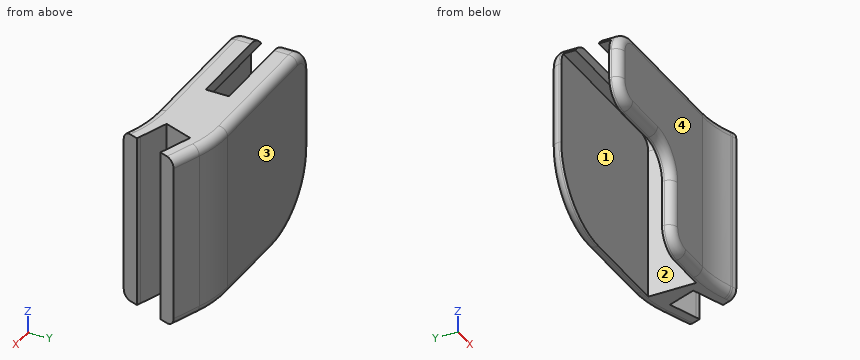
```python
from build123d import *

# Parameters (mm, degrees)
F0_W         = 30
F0_H         = 12
F1_DEPTH     = 30
F2_W         = 8.215
F2_H         = 28.15
F3_DEPTH     = 28
F4_W         = 5.3
F4_H         = 30
F5_DEPTH     = 5.3
F6_W         = 17
F6_H         = 17
F7_DEPTH     = 2.8
F8_DEPTH     = 0.75
F9_R         = 12
F10_T1_DEPTH = 32
F10_T3_DEPTH = 11.8925
F11_R        = 20
F12_R        = 5
F13_R        = 1.5
F14_R        = 2
F15_W        = 5.0863461345
F15_H        = 4
F15_W_2      = 14.4734603858
F16_DEPTH    = 30.0010001


# Not quite as in the source:
# - a fillet or chamfer that OpenCascade refuses, or shapes differently, is made with other operations: its cross-section is extruded or revolved along the edge and cut away or added


with BuildPart() as f1:
    # F0 (on Top) → F1 (new body)
    with BuildSketch(Plane.XY):
        with Locations((-15, 6)):
            Rectangle(F0_W, F0_H)
        Polygon((0, 12), (0, 0), (3.6608153082, -1.3324278053), (7.5175409663, 9.2638388534), align=None)
    extrude(amount=F1_DEPTH)

    # F2 (on face) → F3 (cut)
    with BuildSketch(Plane(origin=(-30, 0, 0), x_dir=(0, -1, 0), z_dir=(-1, 0, 0))):
        with Locations((-6, 14.075)):
            Rectangle(F2_W, F2_H)
    extrude(amount=-F3_DEPTH, mode=Mode.SUBTRACT)

    # F4 (on face) → F5 (cut)
    with BuildSketch(Plane(origin=(3.6608153082, -1.3324278053, 0), x_dir=(0.3420201433, 0.9396926208, 0), z_dir=(0.9396926208, -0.3420201433, 0))):
        with Locations((5.6381557247, 15)):
            Rectangle(F4_W, F4_H)
    extrude(amount=-F5_DEPTH, mode=Mode.SUBTRACT)

    # F6 (on face) → F7 (cut)
    with BuildSketch(Plane.XZ):
        with Locations((-21.5, 8.5)):
            Rectangle(F6_W, F6_H)
    extrude(amount=-F7_DEPTH, mode=Mode.SUBTRACT)

    # F8 (add): faces of the model
    f8_faces = [f1.faces().sort_by_distance(p)[0] for p in [
        (7.0065362417, 7.8598649113, 15),
        (4.1718200328, 0.0715461368, 15),
    ]]
    extrude(f8_faces, amount=F8_DEPTH)

    # F9
    f9_edges = [f1.edges().sort_by_distance(p)[0] for p in [
        (-30, 11.05375, 0),
    ]]
    fillet(f9_edges, radius=F9_R)

    # F10: fillet of radius 4 on 3 edges, made by hand

    # F10_s2 → F10_t1 (cut)
    with BuildSketch(Plane.XZ.offset(-22)):
        with BuildLine():
            ThreePointArc((-30, 26), (-28.8284271247, 28.8284271247), (-26, 30))
            Line((-26, 30), (-30, 30))
            Line((-30, 30), (-30, 26))
        make_face()
    extrude(amount=F10_T1_DEPTH, mode=Mode.SUBTRACT)

    # F10_s4 → F10_t3 (cut)
    with BuildSketch(Plane.XZ.offset(-1.8925)):
        with BuildLine():
            ThreePointArc((-30, 21), (-28.8284271247, 18.1715728753), (-26, 17))
            Line((-26, 17), (-30, 17))
            Line((-30, 17), (-30, 21))
        make_face()
        with BuildLine():
            ThreePointArc((-9, 0), (-11.8284271247, 1.1715728753), (-13, 4))
            Line((-13, 4), (-13, 0))
            Line((-13, 0), (-9, 0))
        make_face()
    extrude(amount=F10_T3_DEPTH, mode=Mode.SUBTRACT)

    # F11
    f11_edges = [f1.edges().sort_by_distance(p)[0] for p in [
        (0, 12, 15),
        (0, 0, 15),
    ]]
    fillet(f11_edges, radius=F11_R)

    # F12
    f12_edges = [f1.edges().sort_by_distance(p)[0] for p in [
        (-13, 0.94625, 17),
    ]]
    fillet(f12_edges, radius=F12_R)

    # F13
    f13_edges = [f1.edges().sort_by_distance(p)[0] for p in [
        (-14.464466, 0, 15.535534),
        (-22, 0, 17),
        (-28.828427, 0, 28.828427),
        (-14.76327, 0, 30),
        (-0.053576, -0.303845, 30),
        (3.839724, -1.397545, 30),
        (3.839724, -1.397545, 0),
        (-0.053576, -0.303845, 0),
        (-6.26327, 0, 0),
        (-11.828427, 0, 1.171573),
        (-13, 0, 8),
        (-14.76327, 12, 30),
        (-0.053576, 11.696155, 30),
        (-28.828427, 0, 18.171573),
        (-30, 0, 23.5),
        (-10.76327, 12, 0),
        (-0.053576, 11.696155, 0),
        (5.768087, 9.900588, 0),
        (5.768087, 9.900588, 30),
        (-28.828427, 12, 28.828427),
        (-30, 12, 19),
        (-26.485281, 12, 3.514719),
    ]]
    fillet(f13_edges, radius=F13_R)

    # F14
    f14_edges = [f1.edges().sort_by_distance(p)[0] for p in [
        (-2, 6, 28.15),
    ]]
    fillet(f14_edges, radius=F14_R)

    # F15 (on face) → F16 (cut, through all)
    with BuildSketch(Plane.XY.offset(30)):
        with Locations((-28.5431730673, 6)):
            Rectangle(F15_W, F15_H)
        with Locations((-18.7632698071, 6)):
            Rectangle(F15_W_2, F15_H)
    extrude(amount=-F16_DEPTH, mode=Mode.SUBTRACT)


solid = f1.part
```
The listing builds one solid part. Answer for the finished solid, in the listing's coordinates (mm). Face numbers are marked on the shaded views. Coordinates: 2 decimals unless noted, no trailing zeros. Loops run counter-clockwise (first coordinate to the right, second up) from the corner with the lowest first, then second, coordinate; pieces in that order, holes last. Notation, with made-up numbers: M 19.5,8 L 62.5,8 A28 ccw 62.5,37 Z; hole C -21,2.5 d1. An arc over 180 degrees is marked long. Answer as a JSON object with one key per item and string values. Group by question number.
Item 1: Section B-B (x = -5.5) is taken. Write down the section's boundary in (y, z), and give its area (3 significant figures).
Item 2: Determine the mould class of the marked faces 1, 2, 3 and 4 for opening direction Y: +Y half, -Y half, draft (parallel to the pull), parting line (faces both ways), or undercut.
Item 3: Section C-C (y = 2.5) is taken. Write down the section's boundary in (x, z), and give its area (3 significant figures).
Item 4: Section A-A (z = 22.5) is taken. Write down the section's boundary in (x, y).
Item 5: Consider L1, parallel to Y at x = -15.5, z = 26; L2, parallel to Y at x = -11.5, z = 2; L3, parallel to Z at x = -17.5, y = 9.5. Determine where each line is inside the solid, lowest interval first.
Item 6: Section D-D (y = 4.75) is taken. Write down the section's boundary in (x, z), and give its area (3 significant figures).
Item 7: Each of these flat-tipped pins is pushed along its axis until it touches: P1, Ø8, axis at x = -18.5, z = 18, coming from the -Y side; P2, Ø6, axis at y = 1.5, z = 23.5, coming from the +X side; P3, Ø5, axis at x = -23.5, z = 4.5, coming from the -Y side. Where does it stop, or does it pass through?
Solved:
{
 "1": {"outline": "M 0,1.5 A1.5 ccw 1.5,0 L 1.89,0 L 1.89,28.15 L 10.11,28.15 L 10.11,0 L 10.5,0 A1.5 ccw 12,1.5 L 12,28.5 A1.5 ccw 10.5,30 L 1.5,30 A1.5 ccw 0,28.5 Z", "area": "127 mm2"},
 "2": {"face 1": "undercut", "face 2": "undercut", "face 3": "+Y half", "face 4": "-Y half"},
 "3": {"outline": "M -29.37,28.15 L -4,28.15 A2 cw -2,26.15 L -2,0 L 1.87,0 L 1.87,30 L -26,30 A4 ccw Z", "area": "166 mm2"},
 "4": {"outline": "M -30,1.5 A1.5 ccw -28.5,0 L -3.53,0 A20 cw 3.31,-1.21 L 4.37,-1.59 L 5.39,1.22 L -0.3,3.29 L 1.52,8.27 L 7.2,6.2 L 8.22,9.01 L 3.31,10.79 A20 ccw -3.53,12 L -28.5,12 A1.5 ccw -30,10.5 L -30,10.11 L -2,10.11 L -2,1.89 L -30,1.89 Z"},
 "5": {"L1": "y = 0 to 1.89, 10.11 to 12", "L2": "y = 0.17 to 1.89, 10.11 to 12", "L3": "z = 28.15 to 30"},
 "6": {"outline": "M -11.53,28.15 L -4,28.15 A2 cw -2,26.15 L -2,0 L 0.23,0 L 0.23,30 L -11.53,30 Z", "area": "85.5 mm2"},
 "7": {"P1": "stops at y = 0", "P2": "stops at x = 5.39", "P3": "stops at y = 10.11"}
}
